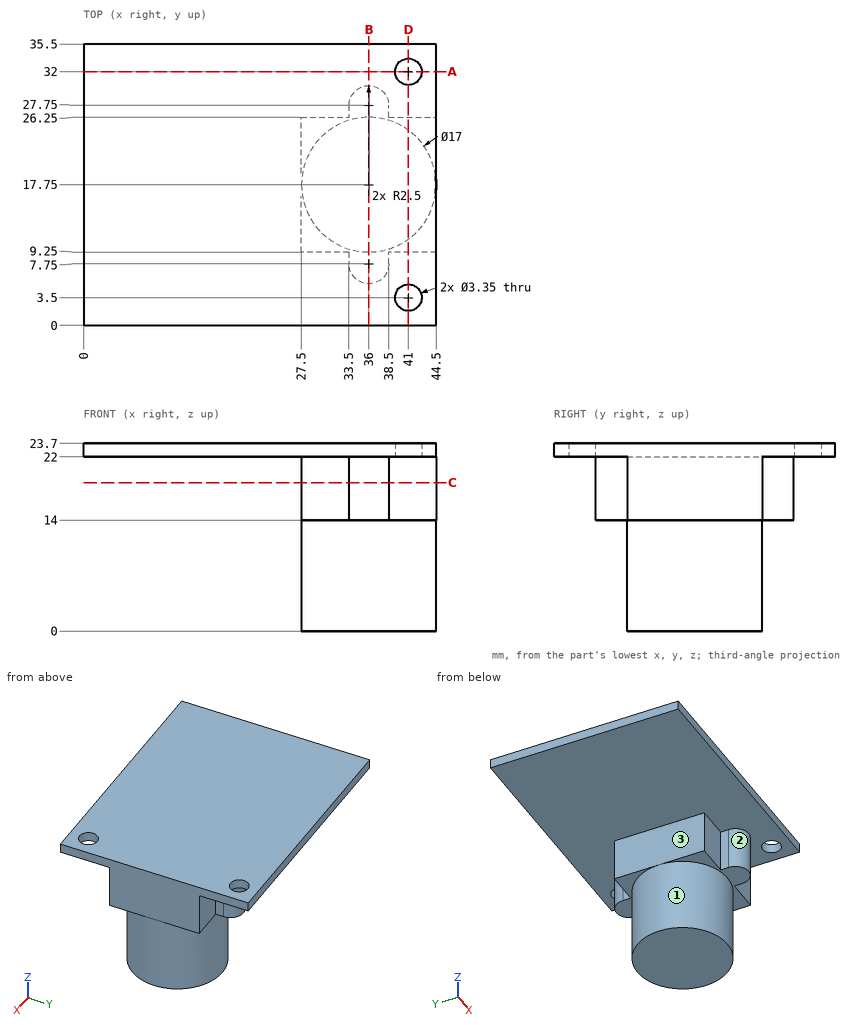
Here's the drawing with two shaded views (mm, measured from the low corner). I have some questions. A direction names the side the tool comes from. Coordinates: 2 decimals unless noted, no trailing zeros. Loops run counter-clockwise (first coordinate to the right, second up) from the corner with the lowest first, then second, coordinate; pieces in that order, holes last. Notation, with made-up numbers: (81, -23.75) -> (128, -23.75) arc R7 ccw to (128, -14.75) -> close; hole circle Ø1 at (53.5, 1.5). An arc over 180 degrees is marked (long way). Answer in a Markdown table with one row per item.
(1) Imagine slicing it at A-A (y = 32). List the corners of the cut face in (x, z) for me (3 decimals).
Results found:
| item | result |
|---|---|
| outline | (0, 22) -> (39.325, 22) -> (39.325, 23.7) -> (0, 23.7) -> close; (42.675, 22) -> (44.5, 22) -> (44.5, 23.7) -> (42.675, 23.7) -> close |
(2) Imagine slicing it at C-C (z = 18.75). List the corners of the cut face in (x, y) for me.
Results found:
| item | result |
|---|---|
| outline | (27.5, 9.25) -> (33.5, 9.25) -> (33.5, 7.75) arc R2.5 ccw to (38.5, 7.75) -> (38.5, 9.25) -> (44.5, 9.25) -> (44.5, 26.25) -> (38.5, 26.25) -> (38.5, 27.75) arc R2.5 ccw to (33.5, 27.75) -> (33.5, 26.25) -> (27.5, 26.25) -> close |
(3) If I drill on probe 1 along X at (y, z) = (32, 22.85) (3 decimals); probe 2 along Y at (x, z) = (41, 23) (3 decimals); probe 3 along Z at (x, y) = (29.5, 4), over which ranges is the centre line in solid material (lowest first)?
Results found:
| item | result |
|---|---|
| probe 1 | x = 0 to 39.325, 42.675 to 44.5 |
| probe 2 | y = 0 to 1.825, 5.175 to 30.325, 33.675 to 35.5 |
| probe 3 | z = 22 to 23.7 |
(4) Will these pins go through, and if not, where does the flat tip stop? pin 1 Ø0.8 at (y, z) = (27, 16.5) entering from -X; pin 2 Ø3 at (x, y) = (6, 24.5) entering from -Z; pin 3 Ø5.5 at (x, y) = (41, 32) entering from +Z; pin 4 Ø0.8 at (y, z) = (8.5, 20) entering from +X.
Results found:
| item | result |
|---|---|
| pin 1 | stops at x = 33.5 |
| pin 2 | stops at z = 22 |
| pin 3 | stops at z = 23.7 |
| pin 4 | stops at x = 38.5 |
(5) For the marked faces 1, 2 and 3, which set-ups out of +Z, -Z, +X, -X, +Y, -Y let a thin tool reach every point of the face, with its end or its side?
Results found:
| item | result |
|---|---|
| face 1 | -Z |
| face 2 | -Z, -Y |
| face 3 | -Z, -X, +Y, -Y |
(6) Imagine slicing it at B-B (x = 36). List the corners of the cut face in (y, z) for me, plus the area to 3 significant figures.
Results found:
| item | result |
|---|---|
| outline | (0, 22) -> (5.25, 22) -> (5.25, 14) -> (9.25, 14) -> (9.25, 0) -> (26.25, 0) -> (26.25, 14) -> (30.25, 14) -> (30.25, 22) -> (35.5, 22) -> (35.5, 23.7) -> (0, 23.7) -> close |
| area | 498 mm^2 |
(7) Imagine slicing it at D-D (x = 41). List the corners of the cut face in (y, z) for me (3 decimals), plus the area to 3 significant figures.
Results found:
| item | result |
|---|---|
| outline | (0, 22) -> (1.825, 22) -> (1.825, 23.7) -> (0, 23.7) -> close; (5.175, 22) -> (9.25, 22) -> (9.25, 14) -> (10.876, 14) -> (10.876, 0) -> (24.624, 0) -> (24.624, 14) -> (26.25, 14) -> (26.25, 22) -> (30.325, 22) -> (30.325, 23.7) -> (5.175, 23.7) -> close; (33.675, 22) -> (35.5, 22) -> (35.5, 23.7) -> (33.675, 23.7) -> close |
| area | 377 mm^2 |
